from build123d import *

# Parameters (mm, degrees)
F3_DEPTH = 22
F4_R     = 30
F5_DEPTH = 25


with BuildPart() as f3:
    # F2 (on Top) → F3 (new body)
    with BuildSketch(Plane.XY):
        with BuildLine():
            Line((23.25, -7.5), (23.25, 7.5))
            ThreePointArc((23.25, 7.5), (0, 30.75), (-23.25, 7.5))
            Line((-23.25, 7.5), (-23.25, -7.5))
            ThreePointArc((-23.25, -7.5), (0, -30.75), (23.25, -7.5))
        make_face()
    extrude(amount=F3_DEPTH)


with BuildPart() as f5:
    # F4 (on face) → F5 (new body)
    with BuildSketch(Plane.XY.offset(22)):
        Circle(F4_R)
    extrude(amount=-F5_DEPTH)

    # F6: intersect F3
    add(f3.part, mode=Mode.INTERSECT)


solid = f5.part
Geometry check sheet. Reference: the model listing, model coordinates, mm. Give positions to 0.01 mm unless a question says otherwise; leave off trailing zeros. Order: outer loops, then holes, each group sorted by start corner. A loop starts at its lowest first (then second) coordinate and runs counter-clockwise, first axis right, second up. Notation, with made-up numbers: (3, -36) - (33, -36) arc R25 cw to (33, -10) - close; hole circle Ø7 at (49.5, 84). An arc over 180 degrees is marked (long way). Use one line per item in the form item = value.
1) Sectioned sample at A-A (z = 2.75). Record the boundary of the cut face in (x, y).
Working result:
outline = (-23.25, -7.5) arc R23.25 ccw to (-11.49, -27.71) arc R30 ccw to (11.49, -27.71) arc R23.25 ccw to (23.25, -7.5) - (23.25, 7.5) arc R23.25 ccw to (11.49, 27.71) arc R30 ccw to (-11.49, 27.71) arc R23.25 ccw to (-23.25, 7.5) - close
2) Sectioned sample at C-C (y = -12.5). Record the boundary of the cut face in (x, z).
Working result:
outline = (-22.71, 0) - (22.71, 0) - (22.71, 22) - (-22.71, 22) - close
3) Sectioned sample at B-B (x = -8). Record the boundary of the cut face in (y, z), and give its area (3 significant figures).
Working result:
outline = (-28.91, 0) - (28.91, 0) - (28.91, 22) - (-28.91, 22) - close
area = 1,270 mm^2
4) Material ranges on probe 1 along Y at (x, z) = (-4, 18.75); probe 2 along Y at (x, z) = (-1.5, 2.75); probe 3 along X at (y, z) = (10.5, 20), recorded low to high. Write a range as from..to.
Working result:
probe_1 = -29.73..29.73
probe_2 = -29.96..29.96
probe_3 = -23.06..23.06
5) Depth check by flat-ended pin: pin 1 Ø2 at (y, z) = (-11, 16) entering from +X; pin 2 Ø4 at (y, z) = (-11.5, 14) entering from +X; pin 3 Ø5 at (x, z) = (-6.5, 17.5) entering from +Y. Enter the tip coordinate at first touch or a pass-through.
Working result:
pin_1 = 23.12
pin_2 = 23.16
pin_3 = 29.73
